```python
from build123d import *

# Parameters (mm, degrees)
SKETCH_1_W             = 90
SKETCH_1_H             = 45
EXTRUDE_1_DEPTH        = 12
HOLE_WIZARD_M121_D     = 10.2
HOLE_WIZARD_M121_DEPTH = 12


with BuildPart() as part:
    # Эскиз1 → Бобышка-Вытянуть1 (new body)
    with BuildSketch(Plane(origin=(0, 0, 0), x_dir=(1, 0, 0), z_dir=(0, 1, 0))):
        Rectangle(SKETCH_1_W, SKETCH_1_H)
    extrude(amount=EXTRUDE_1_DEPTH)

    # Эскиз2 → Вырез-Повернуть1 (revolve, cut)
    with BuildSketch(Plane.XY):
        Polygon((-32.5, 12), (-32.5, 3), (-28, 3), (-28, 0), (-22.5, 0), (-22.5, 12), align=None)
    cut_revolve_1 = revolve(axis=Axis((-22.5, 12, 0), (0, -1, 0)), mode=Mode.SUBTRACT)

    # Зеркальное отражение1: Вырез-Повернуть1 across plane
    add(cut_revolve_1.mirror(Plane(origin=(0, 0, 0), x_dir=(0, 0, 1), z_dir=(1, 0, 0))), mode=Mode.SUBTRACT)

    # Отверстие обработанное метчиком M121
    with Locations(Plane(origin=(0, 12, 0), x_dir=(1, 0, 0), z_dir=(0, 1, 0))):
        with Locations((0, 0)):
            Hole(HOLE_WIZARD_M121_D / 2, depth=HOLE_WIZARD_M121_DEPTH)


solid = part.part
```
Part model, mm, in its own coordinate system. A direction names the side the tool comes from. Round coordinates to 2 decimals unless told otherwise and drop trailing zeros. Loops run counter-clockwise (first coordinate to the right, second up) from the corner with the lowest first, then second, coordinate; pieces in that order, holes last.
1. Slice it at C-C (z = -7). Give the cut face in (x, y), and give its area (3 significant figures).
Solutions:
outline: (-45, 0) - (45, 0) - (45, 12) - (29.64, 12) - (29.64, 3) - (15.36, 3) - (15.36, 12) - (-15.36, 12) - (-15.36, 3) - (-29.64, 3) - (-29.64, 12) - (-45, 12) - close
area: 823 mm2
2. Drill centre lines: line 1 along X through (y, z) = (5.25, 9); line 2 along X through (y, z) = (10.5, -3.5); line 3 along Z through (x, y) = (22.5, 3.5). Where is each one in solid material? Low to high.
Solutions:
line 1: x = -45 to -26.86, -18.14 to 18.14, 26.86 to 45
line 2: x = -45 to -31.87, -13.13 to -3.71, 3.71 to 13.13, 31.87 to 45
line 3: z = -22.5 to -10, 10 to 22.5
3. Two-plate mould, pull along Z, no slides. Class faces 3 (the face through (-45, 6, 0)), 4 (the face through (-27.58, 1.48, 2.11)), 5 (the face through (-1, 6, 22.5)): pulls with the +Z half, pulls with the -Z half, needs draft (parallel to the pull), parting line crosses it, or undercut.
Solutions:
face 3: needs draft
face 4: undercut
face 5: pulls with the +Z half
4. 3-axis set-ups, long thin cutter, end or side, ignore diameter. For faces 1 (the face through (-0.6, 12, -5.3)), 2 (the face through (-32.04, 7.44, -3)): which of +Z, -Z, +X, -X, +Y, -Y reach the whole face in a straight line?
Solutions:
face 1: +Z, -Z, +X, -X, +Y
face 2: +Y
5. Slice it at A-A (x = 0). Give the cut face in (y, z).
Solutions:
outline: (0, -22.5) - (12, -22.5) - (12, -5.1) - (0, -5.1) - close; (0, 5.1) - (12, 5.1) - (12, 22.5) - (0, 22.5) - close
6. Flat gauge pin, fed straight in: pin 1 (6 mm diameter, centred on x = 27, z = 3, fed in from +Y). Where does the tip first touch, or does it go through?
Solutions:
pin 1: stops at y = 3
7. Slice it at B-B (y = 8.25). Give the cut face in (x, z).
Solutions:
outline: (-45, -22.5) - (45, -22.5) - (45, 22.5) - (-45, 22.5) - close; hole circle Ø20 at (-22.5, 0); hole circle Ø10.2 at (0, 0); hole circle Ø20 at (22.5, 0)
8. Slice it at D-D (x = 22.5). Give the cut face in (y, z), and give its area (3 significant figures).
Solutions:
outline: (0, -22.5) - (12, -22.5) - (12, -10) - (3, -10) - (3, -5.5) - (0, -5.5) - close; (0, 5.5) - (3, 5.5) - (3, 10) - (12, 10) - (12, 22.5) - (0, 22.5) - close
area: 327 mm2
